Check sheet for the modelled part. Datum: model origin and axes. Units: mm. A direction names the side the tool comes from. Coordinates: 2 decimals unless noted, no trailing zeros. Loops run counter-clockwise (first coordinate to the right, second up) from the corner with the lowest first, then second, coordinate; pieces in that order, holes last. Notation, with made-up numbers: M 50.25,-2 L 86.25,-2 A6 ccw 86.25,3 Z; hole C -11.75,-17.75 d11. An arc over 180 degrees is marked long. Answer in a Markdown table with one row per item. Add a question column.
```python
from build123d import *

# Parameters (mm, degrees)
SKETCH3_W           = 100
SKETCH3_H           = 1500
BOSS_EXTRUDE2_DEPTH = 70
CUT_EXTRUDE2_DEPTH  = 50


with BuildPart() as part:
    # Sketch3 → Boss-Extrude2 (new body)
    with BuildSketch(Plane(origin=(0, 0, 0), x_dir=(0, 0, -1), z_dir=(1, 0, 0))):
        Rectangle(SKETCH3_W, SKETCH3_H)
    extrude(amount=BOSS_EXTRUDE2_DEPTH)

    # Sketch7 → Cut-Extrude2 (cut)
    with BuildSketch(Plane(origin=(0, 0, 0), x_dir=(0, 0, -1), z_dir=(1, 0, 0))):
        with BuildLine():
            Line((20, 500), (20, -500))
            ThreePointArc((20, -500), (0, -520), (-20, -500))
            Line((-20, -500), (-20, 500))
            ThreePointArc((-20, 500), (0, 520), (20, 500))
        make_face()
    extrude(amount=CUT_EXTRUDE2_DEPTH, mode=Mode.SUBTRACT)


solid = part.part
```
Q1. Cross-section at B-B (y = -206.5). Record the cut outline in (x, z), plus the area to 3 significant figures.
Q2. Go/stop test with a flat-tipped pin: pin 1 (2 mm diameter, centred on y = 481, z = -2, fed in from -X). Record where the tip stops, or that it passes through.
Q3. Cross-section at A-A (x = 12). Record the cut outline in (y, z), plus the area to 3 significant figures.
Q4. Thickness scan on L1, parallel to Z at x = 28, y = 93; L2, parallel to X at y = 377, z = -8.5; L3, parallel to Y at x = 48, z = 14.5. Record the ranges inside material, lowest first.
Q5. Access from +Z, -Z, +X, -X, +Y, -Y to the whole of each face (thin tool, end or side, straight path). Record for faces 4 (the face through (35, 750, 1)), 5 (the face through (25, 520, 0)).
Q6. Mould release check, pull along Z, two halves, no side actions. Record for faces 1 (the face through (0, 10, 23)), 2 (the face through (35, -10, 50)), 3 (the face through (25, 7, -20)): released by +Z, released by -Z, zero draft, split by the parting line, or undercut.
Q7. Cross-section at C-C (z = 0). Record the cut outline in (x, y), plus the area to 3 significant figures.
Answer key:
| question | item | result |
|---|---|---|
| 1 | outline | M 0,-50 L 70,-50 L 70,50 L 0,50 L 0,20 L 50,20 L 50,-20 L 0,-20 Z |
| 1 | area | 5,000 mm^2 |
| 2 | pin 1 | x = 50 |
| 3 | outline | M -750,-50 L 750,-50 L 750,50 L -750,50 Z; hole M -500,-20 L 500,-20 A20 ccw 500,20 L -500,20 A20 ccw Z |
| 3 | area | 109,000 mm^2 |
| 4 | L1 | -50 to -20, 20 to 50 |
| 4 | L2 | 50 to 70 |
| 4 | L3 | -750 to -513.77, 513.77 to 750 |
| 5 | face 4 | +Z, -Z, +X, -X, +Y |
| 5 | face 5 | -X |
| 6 | face 1 | zero draft |
| 6 | face 2 | released by +Z |
| 6 | face 3 | undercut |
| 7 | outline | M 0,-750 L 70,-750 L 70,750 L 0,750 L 0,520 L 50,520 L 50,-520 L 0,-520 Z |
| 7 | area | 53,000 mm^2 |
